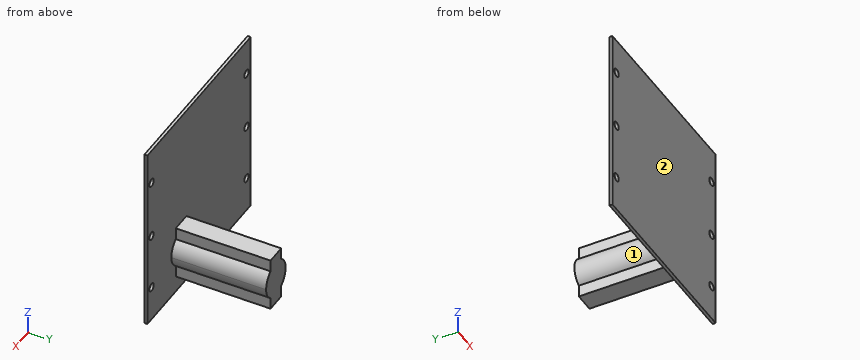
```python
from build123d import *

# Parameters (mm, degrees)
CROQUIS1_W              = 100
CROQUIS1_H              = 100
CROQUIS1_R              = 2.1
SALIENTE_EXTRUIR1_DEPTH = 1.6
SALIENTE_EXTRUIR2_DEPTH = 50


with BuildPart() as part:
    # Croquis1 → Saliente-Extruir1 (new body)
    with BuildSketch(Plane(origin=(0, 0, 0), x_dir=(1, 0, 0), z_dir=(0, 1, 0))):
        Rectangle(CROQUIS1_W, CROQUIS1_H)
        with Locations(Location((-46, 31, 0), (0, 0, 270))):
            Circle(CROQUIS1_R, mode=Mode.SUBTRACT)
        with Locations(Location((-46, 0.5, 0), (0, 0, 270))):
            Circle(CROQUIS1_R, mode=Mode.SUBTRACT)
        with Locations(Location((-46, -31, 0), (0, 0, 270))):
            Circle(CROQUIS1_R, mode=Mode.SUBTRACT)
        with Locations(Location((46, -31, 0), (0, 0, 90))):
            Circle(CROQUIS1_R, mode=Mode.SUBTRACT)
        with Locations(Location((46, 0.5, 0), (0, 0, 90))):
            Circle(CROQUIS1_R, mode=Mode.SUBTRACT)
        with Locations(Location((46, 31, 0), (0, 0, 90))):
            Circle(CROQUIS1_R, mode=Mode.SUBTRACT)
    extrude(amount=SALIENTE_EXTRUIR1_DEPTH)

    # Croquis2 → Saliente-Extruir2 (add)
    with BuildSketch(Plane(origin=(0, 1.6, 0), x_dir=(1, 0, 0), z_dir=(0, 1, 0))):
        with BuildLine():
            Line((12.217414709, 18.903028856), (12.217414709, 34.689006191))
            ThreePointArc((12.217414709, 34.689006191), (7.951157107, 26.796017524), (12.217414709, 18.903028856))
        make_face()
        with BuildLine():
            ThreePointArc((22.553948572, 34.689006191), (17.38568164, 36.230542057), (12.217414709, 34.689006191))
            Line((12.217414709, 34.689006191), (12.217414709, 18.903028856))
            ThreePointArc((12.217414709, 18.903028856), (17.38568164, 17.36149299), (22.553948572, 18.903028856))
            Line((22.553948572, 18.903028856), (22.553948572, 34.689006191))
        make_face()
        with BuildLine():
            Line((22.553948572, 41.084489345), (12.217414709, 41.084489345))
            Line((12.217414709, 41.084489345), (12.217414709, 34.689006191))
            ThreePointArc((12.217414709, 34.689006191), (17.38568164, 36.230542057), (22.553948572, 34.689006191))
            Line((22.553948572, 34.689006191), (22.553948572, 41.084489345))
        make_face()
        with BuildLine():
            ThreePointArc((26.820206174, 26.796017524), (25.685392308, 31.282113377), (22.553948572, 34.689006191))
            Line((22.553948572, 34.689006191), (22.553948572, 18.903028856))
            ThreePointArc((22.553948572, 18.903028856), (25.685392308, 22.30992167), (26.820206174, 26.796017524))
        make_face()
        with BuildLine():
            ThreePointArc((22.553948572, 18.903028856), (17.38568164, 17.36149299), (12.217414709, 18.903028856))
            Line((12.217414709, 18.903028856), (12.217414709, 12.507545702))
            Line((12.217414709, 12.507545702), (22.553948572, 12.507545702))
            Line((22.553948572, 12.507545702), (22.553948572, 18.903028856))
        make_face()
    extrude(amount=SALIENTE_EXTRUIR2_DEPTH)


solid = part.part
```
Model file for the job. Use its own axes, mm. Face numbers are marked on the shaded views. A direction names the side the tool comes from. Coordinates: 2 decimals unless noted, no trailing zeros. Loops run counter-clockwise (first coordinate to the right, second up) from the corner with the lowest first, then second, coordinate; pieces in that order, holes last. Notation, with made-up numbers: M 50,-11.75 L 91,-11.75 A13 ccw 91,13.25 Z; hole C 62.25,-18 d1. An arc over 180 degrees is marked long. Use CSV: the item, a comma, the result in double quotes. Start each with the question number.
1. Flat gauge pins, fed straight in: pin 1 (5 mm diameter, centred on x = 16.5, y = 31, fed in from -Z); pin 2 (5 mm diameter, centred on x = 17.5, y = 29.5, fed in from +Z); pin 3 (3 mm diameter, centred on x = 9.5, y = 28, fed in from +Z); pin 4 (4 mm diameter, centred on x = 46, z = 31, fed in from -Y). Where does each tip first touch, or does it go through?
2. Tool access for the marked faces 1 and 2: list every direction of +Z, -Z, +X, -X, +Y, -Y with a clear straight run to the whole face (end or side of a thin tool).
3. Probe probe 1 along X at (y, z) = (1.2, 31); probe 2 along Y at (x, z) = (-1.5, -7); probe 3 along Z at (x, y) = (14, 15.5). List the from-to ranges inside material, lowest first. Write a range as [from, to].
4. Band-saw the part on A-A, the plane x = 46. List the corners of the cut face in (y, z).
5. Band-saw the part on C-C, the plane y = 26. List the corners of the cut face in (x, z), then the cut area to 3 significant figures.
6. Band-saw the part on D-D, the plane z = -15.5. List the corners of the cut face in (x, y), then the cut area to 3 significant figures.
7. Band-saw the part on B-B, the plane z = -0.5. List the corners of the cut face in (x, y), then the cut area to 3 significant figures.
Entries:
1,pin 1,"stops at z = -41.08"
1,pin 2,"stops at z = -12.51"
1,pin 3,"stops at z = -19.85"
1,pin 4,"passes through"
2,face 1,"-X, +Y"
2,face 2,"+Z, -Z, +X, -X, -Y"
3,probe 1,"x = [-50, -48.1], [-43.9, 43.9], [48.1, 50]"
3,probe 2,"y = [0, 1.6]"
3,probe 3,"z = [-41.08, -12.51]"
4,outline,"M 0,-50 L 1.6,-50 L 1.6,-33.1 L 0,-33.1 Z; M 0,-28.9 L 1.6,-28.9 L 1.6,-2.6 L 0,-2.6 Z; M 0,1.6 L 1.6,1.6 L 1.6,28.9 L 0,28.9 Z; M 0,33.1 L 1.6,33.1 L 1.6,50 L 0,50 Z"
5,outline,"M 12.22,-41.08 L 22.55,-41.08 L 22.55,-34.69 A9.43 ccw 22.55,-18.9 L 22.55,-12.51 L 12.22,-12.51 L 12.22,-18.9 A9.43 ccw 12.22,-34.69 Z"
5,area,"390 mm2"
6,outline,"M -50,0 L 50,0 L 50,1.6 L 22.55,1.6 L 22.55,51.6 L 12.22,51.6 L 12.22,1.6 L -50,1.6 Z"
6,area,"677 mm2"
7,outline,"M -50,0 L -48.1,0 L -48.1,1.6 L -50,1.6 Z; M -43.9,0 L 43.9,0 L 43.9,1.6 L -43.9,1.6 Z; M 48.1,0 L 50,0 L 50,1.6 L 48.1,1.6 Z"
7,area,"147 mm2"
